Work out the finished part from the listing and answer in its coordinate system (mm). Face numbers are marked on the shaded views. Give positions to 0.01 mm unless a question says otherwise; leave off trailing zeros. Order: outer loops, then holes, each group sorted by start corner. A loop starts at its lowest first (then second) coordinate and runs counter-clockwise, first axis right, second up. Notation, with made-up numbers: (-29, 6) - (-1, 6) arc R22 cw to (-1, 37) - close; hole circle Ø10 at (61.5, 76.25). An arc over 180 degrees is marked (long way). Write each question's results on one line, items separated by ' | '.
from build123d import *

# Parameters (mm, degrees)
F0_W     = 273.05
F0_H     = 114.3
F2_DEPTH = 25.4
F1_R     = 37.690445
F1_R_2   = 37.958893
F4_DEPTH = 25.4
F5_DEPTH = 25.4
F6_DEPTH = 25.4
F7_DEPTH = 25.4


with BuildPart() as f2:
    # F0 (on Front) → F2 (new body)
    with BuildSketch(Plane.XZ):
        with Locations((136.525, 57.15)):
            Rectangle(F0_W, F0_H)
    extrude(amount=F2_DEPTH)

    # F1 (on face) → F4 (cut)
    with BuildSketch(Plane.XZ):
        with Locations((49.946755, 50.604541)):
            Circle(F1_R)
        with Locations((224.03121, 50.220247)):
            Circle(F1_R_2)
    extrude(amount=-F4_DEPTH, mode=Mode.SUBTRACT)

    # F1 (on face) → F5 (cut)
    with BuildSketch(Plane.XZ):
        with Locations((49.946755, 50.604541)):
            Circle(F1_R)
        with Locations((224.03121, 50.220247)):
            Circle(F1_R_2)
    extrude(amount=-F5_DEPTH, mode=Mode.SUBTRACT)

    # F1 (on face) → F6 (cut)
    with BuildSketch(Plane.XZ):
        with Locations((49.946755, 50.604541)):
            Circle(F1_R)
        with Locations((224.03121, 50.220247)):
            Circle(F1_R_2)
    extrude(amount=-F6_DEPTH, mode=Mode.SUBTRACT)

    # F1 (on face) → F7 (cut)
    with BuildSketch(Plane.XZ):
        with Locations((49.946755, 50.604541)):
            Circle(F1_R)
        with Locations((224.03121, 50.220247)):
            Circle(F1_R_2)
    extrude(amount=F7_DEPTH, mode=Mode.SUBTRACT)


solid = f2.part
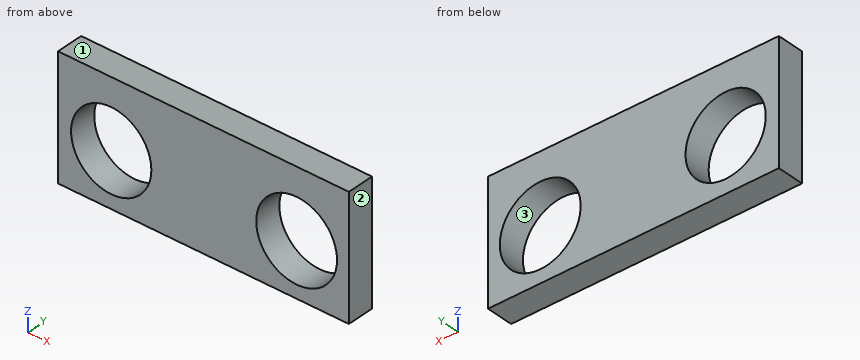
1. Straight lines are drawn through the part: line 1 (Z direction, x = 49, y = -21.5); line 2 (X direction, y = -11, z = 43); line 3 (X direction, y = -21.5, z = 45.5). For each, find the intervals that lie inside material, in ascending order. Write a range as [from, to].
Answer list:
line 1: [0, 12.93], [88.28, 114.3] | line 2: [0, 13.03], [86.86, 186.77], [261.3, 273.05] | line 3: [0, 12.6], [87.29, 186.37], [261.7, 273.05]
2. A cutting plane is placed at C-C, the plane y = -5. Write down the section's boundary in (x, z), then the cut area to 3 significant figures.
Answer list:
outline: (0, 0) - (273.05, 0) - (273.05, 114.3) - (0, 114.3) - close; hole circle Ø75.38 at (49.95, 50.6); hole circle Ø75.92 at (224.03, 50.22) | area: 22,200 mm^2
3. A cutting plane is placed at B-B, the plane x = 22.5. Write down the section's boundary in (y, z).
Answer list:
outline: (-25.4, 0) - (0, 0) - (0, 24.77) - (-25.4, 24.77) - close; (-25.4, 76.44) - (0, 76.44) - (0, 114.3) - (-25.4, 114.3) - close
4. A cutting plane is placed at A-A, the plane z = 81.5. Write down the section's boundary in (x, y), then the cut area to 3 significant figures.
Answer list:
outline: (0, -25.4) - (28.36, -25.4) - (28.36, 0) - (0, 0) - close; (71.53, -25.4) - (202.53, -25.4) - (202.53, 0) - (71.53, 0) - close; (245.54, -25.4) - (273.05, -25.4) - (273.05, 0) - (245.54, 0) - close | area: 4,750 mm^2
5. Determine the mould class of the marked faces 1, 2 and 3 for opening direction X: +X half, -X half, draft (parallel to the pull), parting line (faces both ways), or undercut.
Answer list:
face 1: draft | face 2: +X half | face 3: undercut
6. A cutting plane is placed at D-D, the plane x = 224. Write down the section's boundary in (y, z), then the cut area to 3 significant figures.
Answer list:
outline: (-25.4, 0) - (0, 0) - (0, 12.26) - (-25.4, 12.26) - close; (-25.4, 88.18) - (0, 88.18) - (0, 114.3) - (-25.4, 114.3) - close | area: 975 mm^2
